Check sheet for the modelled part. Datum: model origin and axes. Units: mm. A direction names the side the tool comes from. Give positions to 0.01 mm unless a question says otherwise; leave off trailing zeros. Write each loop counter-clockwise with the first axis right and the second up, starting at its lowest first coordinate (ties: lowest second). Pieces come first, ordered by that corner, then holes. Notation, with made-up numbers: M -19.75,10 L 15.25,10 A22 cw 15.25,49 Z; hole C -6,54.5 d10. An arc over 180 degrees is marked long. Write item = value, one per line. Start each with the question number.
1) Sectioned sample at C-C, the plane y = 1.25. Record the cut outline in (x, z).
2) Set-up check for faces 4 (the face through (1, 2.45, 1)), 5 (the face through (0, 1.45, 0)): record each of +Z, -Z, +X, -X, +Y, -Y from which the full face is reachable in a straight line by a thin tool's end or side.
3) Gauge pin test, flat ends, axial feed: pin 1 (1 mm diameter, centred on y = 2, z = -1, fed in from -X); pin 2 (1.9 mm diameter, centred on x = -0.5, z = 0, fed in from +Y); pin 3 (0.5 mm diameter, centred on x = 0, y = 2, fed in from -Z); pin 4 (0.8 mm diameter, centred on x = 0.5, y = 2, fed in from +Z). Record the tip position at first contact, or that the pin passes through.
4) Draft check along X on faces 1 (the face through (-0.63, 0.15, 2.83)), 2 (the face through (-0.999, 1.957, -0.587)), 3 (the face through (0, 0, 0)). Enter one of: pulls with the +X half, pulls with the -X half, needs draft (parallel to the pull), parting line crosses it, or undercut.
5) Sectioned sample at B-B, the plane x = 0. Record the cut outline in (y, z), then the cut area to 3 significant figures.
6) Sectioned sample at D-D, the plane y = 0.4. Record the cut outline in (x, z), then the cut area to 3 significant figures.
7) Scan lines: L1, parallel to Z at x = -1, y = 2.3; L2, parallel to X at y = 1.5, z = 1; L3, parallel to X at y = 1.9, z = 0.75. Record each from-to range of solid material in increasing order.
8) Sectioned sample at A-A, the plane y = 2.2. Record the cut outline in (x, z).
from build123d import *

# Parameters (mm, degrees)
SKETCH5_R          = 2.75
SKETCH4_R          = 5.2
CUT_EXTRUDE1_DEPTH = 1


with BuildPart() as part:
    # Sketch5 → Loft1 section 0
    with BuildSketch(Plane(origin=(0, 0, 0), x_dir=(1, 0, 0), z_dir=(0, 1, 0))):
        Circle(SKETCH5_R)
    # Sketch4 → Loft1 section 1
    with BuildSketch(Plane(origin=(0, 2.45, 0), x_dir=(1, 0, 0), z_dir=(0, 1, 0))):
        Circle(SKETCH4_R)
    loft()

    # Sketch6 → Cut-Extrude1 (cut)
    with BuildSketch(Plane(origin=(0, 2.45, 0), x_dir=(1, 0, 0), z_dir=(0, 1, 0))):
        Polygon((1.337999459, 0), (0.66899973, 1.158741522), (-0.66899973, 1.158741522), (-1.337999459, 0), (-0.66899973, -1.158741522), (0.66899973, -1.158741522), align=None)
    extrude(amount=-CUT_EXTRUDE1_DEPTH, mode=Mode.SUBTRACT)


solid = part.part
Data:
q1.outline = C 0,0 d8
q2.face_4 = +Z, -Z, +X, -X, +Y
q2.face_5 = +Y
q3.pin_1 = -5.14
q3.pin_2 = 2.45
q3.pin_3 = -5
q3.pin_4 = 5.13
q4.face_1 = parting line crosses it
q4.face_2 = undercut
q4.face_3 = needs draft
q5.outline = M 0,-2.75 L 2.45,-5.2 L 2.45,-1.16 L 1.45,-1.16 L 1.45,1.16 L 2.45,1.16 L 2.45,5.2 L 0,2.75 Z
q5.area = 17.2 mm2
q6.outline = C 0,0 d6.3
q6.area = 31.2 mm2
q7.L1 = -4.95 to -0.59, 0.59 to 4.95
q7.L2 = -4.13 to -0.76, 0.76 to 4.13
q7.L3 = -4.59 to -0.9, 0.9 to 4.59
q8.outline = C 0,0 d9.9; hole M -1.34,0 L -0.67,-1.16 L 0.67,-1.16 L 1.34,0 L 0.67,1.16 L -0.67,1.16 Z
